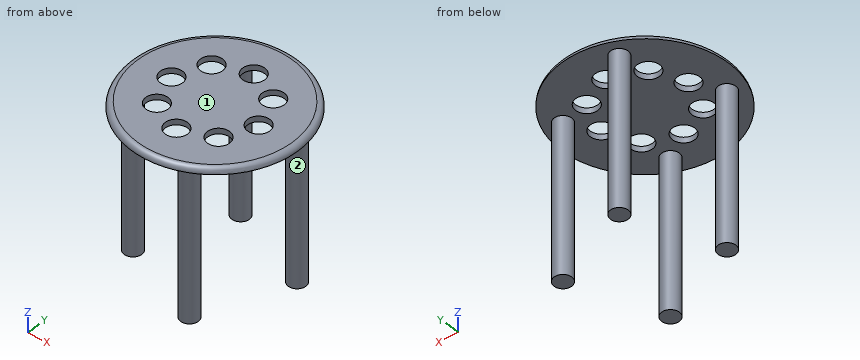
from build123d import *

# Parameters (mm, degrees)
F0_R     = 75
F0_R_2   = 10
F1_DEPTH = 5
F3_R     = 7.9557273046
F4_DEPTH = 139.446


# Not quite as in the source:
# - a fillet or chamfer that OpenCascade refuses, or shapes differently, is made with other operations: its cross-section is extruded or revolved along the edge and cut away or added


with BuildPart() as f1:
    # F0 (on Top) → F1 (new body)
    with BuildSketch(Plane.XY):
        Circle(F0_R)
        with Locations((-28.2842712475, -28.2842712475)):
            Circle(F0_R_2, mode=Mode.SUBTRACT)
        with Locations((0, -40)):
            Circle(F0_R_2, mode=Mode.SUBTRACT)
        with Locations((28.2842712475, -28.2842712475)):
            Circle(F0_R_2, mode=Mode.SUBTRACT)
        with Locations((-40, 0)):
            Circle(F0_R_2, mode=Mode.SUBTRACT)
        with Locations((-28.2842712475, 28.2842712475)):
            Circle(F0_R_2, mode=Mode.SUBTRACT)
        with Locations((28.2842712475, 28.2842712475)):
            Circle(F0_R_2, mode=Mode.SUBTRACT)
        with Locations((40, 0)):
            Circle(F0_R_2, mode=Mode.SUBTRACT)
        with Locations((0, 40)):
            Circle(F0_R_2, mode=Mode.SUBTRACT)
    extrude(amount=F1_DEPTH)

    # F2: fillet of radius 5.08 on 1 edges, made by hand

    # F2_s1 → F2_t2 (revolve, cut)
    with BuildSketch(Plane.XZ):
        with BuildLine():
            ThreePointArc((75, -0.08), (73.5121024484, 3.5121024484), (69.92, 5))
            Line((69.92, 5), (75, 5))
            Line((75, 5), (75, -0.08))
        make_face()
    revolve(axis=Axis((0, 0, 5), (0, 0, 1)), mode=Mode.SUBTRACT)

    # F3 (on Top) → F4 (join)
    with BuildSketch(Plane.XY):
        with Locations((24.1924598813, -53.7772104144)):
            Circle(F3_R)
        with Locations((53.7772104144, 24.1924598813)):
            Circle(F3_R)
        with Locations((-24.1924598813, 53.7772104144)):
            Circle(F3_R)
        with Locations((-53.7772104144, -24.1924598813)):
            Circle(F3_R)
    extrude(amount=-F4_DEPTH)


solid = f1.part
CAD build for the part. Positions are in the model's coordinates, mm. Face numbers are marked on the shaded views. A direction names the side the tool comes from. Give positions to 0.01 mm unless a question says otherwise; leave off trailing zeros. Write each loop counter-clockwise with the first axis right and the second up, starting at its lowest first coordinate (ties: lowest second). Pieces come first, ordered by that corner, then holes. Notation, with made-up numbers: (14.25, 73.5) - (20.25, 73.5) arc R10 cw to (20.25, 85.5) - close; hole circle Ø1 at (-40, 75). An arc over 180 degrees is marked (long way). Answer as CSV lines item,"result".
Q1. Flat gauge pins, fed straight in: pin 1 Ø10 at (y, z) = (-49.5, -70.5) entering from -X; pin 2 Ø3 at (y, z) = (-56.5, -37) entering from +X; pin 3 Ø18 at (x, y) = (28.28, 28.28) entering from -Z; pin 4 Ø1 at (x, z) = (-25.5, -74) entering from +Y. Where does each tip first touch, or does it go through?
Result set:
pin 1,"x = 16.24"
pin 2,"x = 32.05"
pin 3,"through"
pin 4,"y = 61.69"
Q2. Band-saw the part on B-B (z = -98). Give the cut face in (x, y), and give its area (3 significant figures).
Result set:
outline,"circle Ø15.91 at (-53.78, -24.19); circle Ø15.91 at (-24.19, 53.78); circle Ø15.91 at (24.19, -53.78); circle Ø15.91 at (53.78, 24.19)"
area,"795 mm²"
Q3. Band-saw the part on A-A (y = 0). Give the cut face in (x, z).
Result set:
outline,"(-75, 0) - (-50, 0) - (-50, 5) - (-69.92, 5) arc R5.08 ccw to start; (-30, 0) - (30, 0) - (30, 5) - (-30, 5) - close; (50, 0) - (75, 0) arc R5.08 ccw to (69.92, 5) - (50, 5) - close"
Q4. 3-axis set-ups, long thin cutter, end or side, ignore diameter. For the marked faces 1 and 2: which of +Z, -Z, +X, -X, +Y, -Y reach the whole face in a straight line?
Result set:
face 1,"+Z, +X, -X, +Y, -Y"
face 2,"-Z"
Q5. Drill centre lines: line 1 (Y direction, x = 0, z = 3); line 2 (Z direction, x = 11, y = 63.5); line 3 (Y direction, x = 50, z = -79.5). Where is each one in solid material? Low to high. Write a range as from..to.
Result set:
line 1,"-73.96..-50, -30..30, 50..73.96"
line 2,"0..5"
line 3,"17.19..31.19"
